Design review of the part built by this model. Coordinates are the model's own, in mm. A direction names the side the tool comes from. Coordinates: 2 decimals unless noted, no trailing zeros. Write each loop counter-clockwise with the first axis right and the second up, starting at its lowest first coordinate (ties: lowest second). Pieces come first, ordered by that corner, then holes. Notation, with made-up numbers: (50.5, 31) -> (69.5, 31) arc R23 cw to (69.5, 61) -> close; hole circle Ø11 at (10.5, 54.25). An arc over 180 degrees is marked (long way). Return JSON: item names as keys, results as strings. Group by question number.
from build123d import *

# Parameters (mm, degrees)
BOSS_EXTRUDE1_START = 2.6
BOSS_EXTRUDE1_DEPTH = 7
CUT_EXTRUDE1_START  = -0.8
CUT_EXTRUDE1_DEPTH  = 10
SKETCH3_R           = 1.75
CUT_EXTRUDE2_DEPTH  = 5


with BuildPart() as part:
    # Sketch1 → Boss-Extrude1 (new, symmetric)
    with BuildSketch(Plane(origin=(0, 887.368143731, 0), x_dir=(1, 0, 0), z_dir=(0, 1, 0)).offset(BOSS_EXTRUDE1_START)):
        with BuildLine():
            Line((633.443700104, -1269.972215541), (633.443700891, -1272.141337124))
            ThreePointArc((633.443700891, -1272.141337124), (633.869649439, -1272.778813799), (634.62160457, -1272.629240553))
            Line((634.62160457, -1272.629240553), (636.9613816, -1270.289463523))
            ThreePointArc((636.9613816, -1270.289463523), (637.592190307, -1269.345391575), (637.813700867, -1268.231782784))
            Line((637.813700867, -1268.231782784), (637.813700862, -1265.982648565))
            ThreePointArc((637.813700862, -1265.982648565), (637.5921903, -1264.86903978), (636.961381595, -1263.924967838))
            Line((636.961381595, -1263.924967838), (634.621604564, -1261.585190807))
            ThreePointArc((634.621604564, -1261.585190807), (633.869649432, -1261.435617561), (633.443700885, -1262.073094238))
            Line((633.443700885, -1262.073094238), (633.443700104, -1264.242215823))
            Line((633.443700104, -1264.242215823), (633.443700104, -1269.972215541))
        make_face()
    extrude(amount=BOSS_EXTRUDE1_DEPTH, both=True)

    # Sketch2 → Cut-Extrude1 (cut)
    with BuildSketch(Plane.ZY.offset(-633.493700104).offset(CUT_EXTRUDE1_START)):
        Polygon((1268.73001891, 887.288143731), (1268.795260282, 887.4011451), (1270.343712913, 890.083143731), (1268.73001891, 892.878143731), (1265.502630906, 892.878143731), (1265.437389534, 892.765142361), (1263.888936903, 890.083143731), (1265.502630906, 887.288143731), align=None)
    extrude(amount=-CUT_EXTRUDE1_DEPTH, mode=Mode.SUBTRACT)

    # Sketch3 → Cut-Extrude2 (cut, symmetric)
    with BuildSketch(Plane.ZY.offset(-633.493700104)):
        with Locations((1267.116324916, 890.083143731)):
            Circle(SKETCH3_R)
    extrude(amount=CUT_EXTRUDE2_DEPTH, both=True, mode=Mode.SUBTRACT)


solid = part.part
Q1. We need section B-B on x = 636.75. Write out the cut boundary in (y, z).
Q2. Wall thickness on L1, parallel to Y at x = 635.45, z = 1268.25; L2, parallel to Z at x = 634.1, y = 890; L3, parallel to Z at x = 637.1, y = 891.5: over which ranges is each line inside the solid? List them lowest first.
Q3. We need section D-D on y = 889.5. Write out the cut boundary in (x, z).
Q4. We need section A-A on y = 887. Write out the cut boundary in (x, z).
Q5. For faces 4 (the flat face through (635.775, 890.066, 1271.476)), 5 (the flat face through (636.01, 891.46, 1269.55)), list the 3-axis set-ups (+Z, -Z, +X, -X, +Y, -Y) from which the entire face can be reached by the end or side of a thin tool; tool diameter is ignored.
Q6. We need section C-C on z = 1268.5. Write out the cut boundary in (x, y), plus the area to 3 significant figures.
Q7. For P1, Ø4.5, axis at y = 890, z = 1267, coming from the +X side; P2, Ø3, axis at y = 890.08, z = 1267.12, coming from the -X side (1 decimal), all flat-tipped, find the tip position at first contact; note any pin that passes through.
Q8. The part is to be moulded in two halves that separate along Z. For faces 1 (the flat face through (634.294, 891, 1269)), 2 (the flat face through (635, 882.968, 1267)), 3 (the cylindrical face through (633.88, 890.07, 1261.43)), say which applies: +Z half, -Z half, draft (parallel to the pull), parting line (faces both ways), or undercut.
Findings below:
{
 "1": {"outline": "(882.97, 1263.71) -> (896.97, 1263.71) -> (896.97, 1270.5) -> (882.97, 1270.5) -> close; hole (887.29, 1265.5) -> (890.08, 1263.89) -> (892.88, 1265.5) -> (892.88, 1268.73) -> (890.08, 1270.34) -> (887.29, 1268.73) -> close"},
 "2": {"L1": "y = 882.97 to 887.29, 892.88 to 896.97", "L2": "z = 1261.38 to 1265.37, 1268.86 to 1272.83", "L3": "z = 1264.07 to 1264.71, 1269.53 to 1270.14"},
 "3": {"outline": "(633.44, 1262.07) arc R0.69 ccw to (634.62, 1261.59) -> (636.96, 1263.92) arc R2.91 ccw to (637.22, 1264.23) -> (634.29, 1264.23) -> (634.29, 1265.47) -> (633.44, 1265.47) -> (633.44, 1264.24) -> close; (633.44, 1268.77) -> (634.29, 1268.77) -> (634.29, 1270.01) -> (637.21, 1270.01) arc R2.91 ccw to (636.96, 1270.29) -> (634.62, 1272.63) arc R0.69 ccw to (633.44, 1272.14) -> (633.44, 1269.97) -> close"},
 "4": {"outline": "(633.44, 1262.07) arc R0.69 ccw to (634.62, 1261.59) -> (636.96, 1263.92) arc R2.91 ccw to (637.81, 1265.98) -> (637.81, 1268.23) arc R2.91 ccw to (636.96, 1270.29) -> (634.62, 1272.63) arc R0.69 ccw to (633.44, 1272.14) -> (633.44, 1269.97) -> (633.44, 1264.24) -> close"},
 "5": {"face 4": "+Z, +X, +Y, -Y", "face 5": "+X"},
 "6": {"outline": "(633.44, 882.97) -> (637.8, 882.97) -> (637.8, 887.29) -> (634.29, 887.29) -> (634.29, 889.01) -> (633.44, 889.01) -> close; (633.44, 891.15) -> (634.29, 891.15) -> (634.29, 892.88) -> (637.8, 892.88) -> (637.8, 896.97) -> (633.44, 896.97) -> close", "area": "39.6 mm^2"},
 "7": {"P1": "stops at x = 634.29", "P2": "passes through"},
 "8": {"face 1": "undercut", "face 2": "draft", "face 3": "-Z half"}
}
